CAD build for the part. Positions are in the model's coordinates, mm. Face numbers are marked on the shaded views. A direction names the side the tool comes from. Give positions to 0.01 mm unless a question says otherwise; leave off trailing zeros. Order: outer loops, then holes, each group sorted by start corner. A loop starts at its lowest first (then second) coordinate and runs counter-clockwise, first axis right, second up.
Item 1: Band-saw the part on D-D on z = -1.5. Give the cut face in (x, y).
Item 2: Which spindle directions (+Z, -Z, +X, -X, +Y, -Y) get a long thin tool onto all of the face, cutting with end or side? Do the marked faces 1 and 2. Say none if no direction does.
Item 3: Two-plate mould, pull along X, no slides. Class the marked faces 3, 4, 5 and 6: released by +X, released by -X, zero draft, split by the parting line, or undercut.
Item 4: Flat gauge pins, fed straight in: P1, Ø2, axis at x = -5.5, z = 4, coming from the +Y side; P2, Ø9.5, axis at x = 2, y = -2.5, coming from the +Z side; P3, Ø4, axis at y = 7, z = 3.5, coming from the -X side. Where does each tip first touch, or does it go through?
Item 5: Band-saw the part on A-A on x = 0. Give the cut face in (y, z), plus the area to 3 significant figures.
Item 6: Band-saw the part on C-C on z = 2.5. Give the cut face in (x, y), plus the area to 3 significant figures.
Item 7: Wall check: L1, parallel to Y at x = 0, z = 3; L2, parallel to Z at x = -2, y = 2.75. Give the ranges that are in metal, low to high.
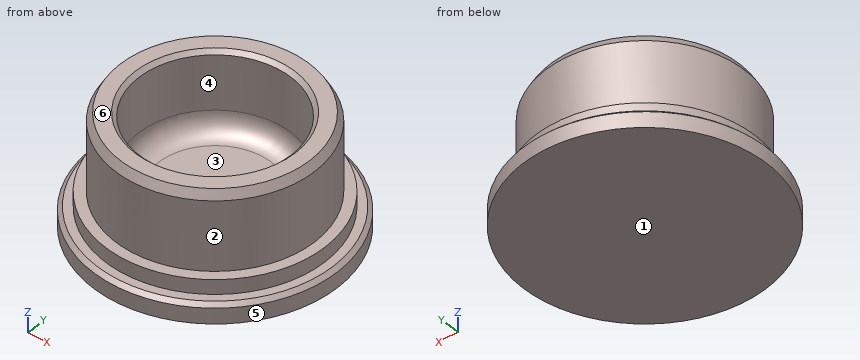
```python
from build123d import *

# Parameters (mm, degrees)
F2_R     = 2
F3_SIZE  = 0.4
F4_SIZE2 = 0.5
F4_SIZE  = 0.8660254038
F5_SIZE  = 0.4


with BuildPart() as f1:
    # F0 (on Front) → F1 (revolve)
    with BuildSketch(Plane.XZ):
        Polygon((10.2, 5.8181819119), (7.8, 5.8181819119), (7.8, -2.1818180881), (0, -2.1818180881), (0, -5.6818180881), (12.5, -5.6818180881), (12.5, -3.6818180881), (11.25, -3.6818180881), (11.25, -2.1818180881), (10.2, -2.1818180881), align=None)
    revolve(axis=Axis((0, 0, 1.239669376), (0, 0, -1)))

    # F2
    f2_edges = [f1.edges().sort_by_distance(p)[0] for p in [
        (-7.8, 0, -2.181818),
    ]]
    fillet(f2_edges, radius=F2_R)

    # F3
    f3_edges = [f1.edges().sort_by_distance(p)[0] for p in [
        (-12.5, 0, -3.681818),
    ]]
    chamfer(f3_edges, length=F3_SIZE)

    # F4
    f4_edges = [f1.edges().sort_by_distance(p)[0] for p in [
        (-10.2, 0, 5.818182),
    ]]
    f4_side = f1.faces().sort_by_distance((-10.2, 0, 1.818182))[0]
    chamfer(f4_edges, length=F4_SIZE, length2=F4_SIZE2, reference=f4_side)

    # F5
    f5_edges = [f1.edges().sort_by_distance(p)[0] for p in [
        (-7.8, 0, 5.818182),
    ]]
    chamfer(f5_edges, length=F5_SIZE)


solid = f1.part
```
The answers:
1. outline: circle Ø20.4 at (0, 0); hole circle Ø14.61 at (0, 0)
2. face 1: -Z, +X, -X, +Y, -Y
2. face 2: +Z
3. face 3: undercut
3. face 4: undercut
3. face 5: split by the parting line
3. face 6: zero draft
4. P1: stops at y = 9.15
4. P2: stops at z = 5.57
4. P3: stops at x = -8.89
5. outline: (-12.5, -5.68) - (12.5, -5.68) - (12.5, -4.08) - (12.1, -3.68) - (11.25, -3.68) - (11.25, -2.18) - (10.2, -2.18) - (10.2, 4.95) - (9.7, 5.82) - (8.2, 5.82) - (7.8, 5.42) - (7.8, -0.18) arc R2 cw to (5.8, -2.18) - (-5.8, -2.18) arc R2 cw to (-7.8, -0.18) - (-7.8, 5.42) - (-8.2, 5.82) - (-9.7, 5.82) - (-10.2, 4.95) - (-10.2, -2.18) - (-11.25, -2.18) - (-11.25, -3.68) - (-12.1, -3.68) - (-12.5, -4.08) - close
5. area: 123 mm2
6. outline: circle Ø20.4 at (0, 0); hole circle Ø15.6 at (0, 0)
6. area: 136 mm2
7. L1: y = -10.2 to -7.8, 7.8 to 10.2
7. L2: z = -5.68 to -2.18
